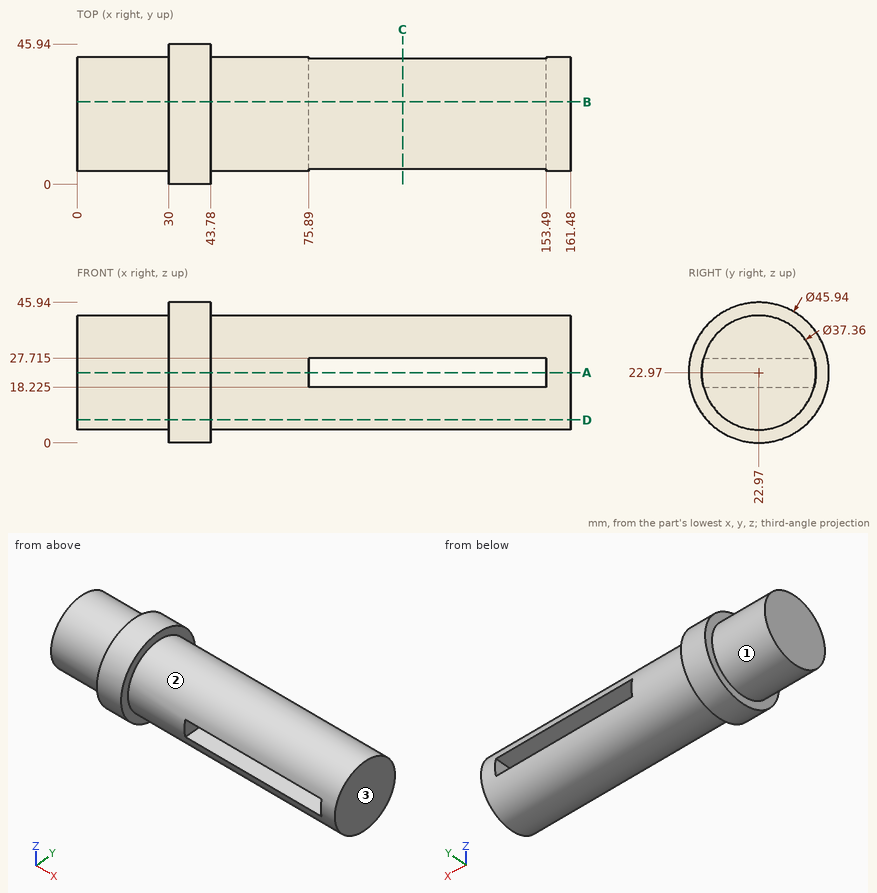
Study the drawing (mm; zero at the part's minimum x, y, z) and answer. A direction names the side the tool comes from. Coordinates: 2 decimals unless noted, no trailing zeros. Write each loop counter-clockwise with the first axis right and the second up, starting at its lowest first coordinate (ties: lowest second). Pieces come first, ordered by that corner, then holes. Notation, with made-up numbers: (38, 24) - (80, 24) arc R14 ccw to (80, 48) - close; hole circle Ø2 at (36, 80.5). An arc over 180 degrees is marked (long way). Answer as a JSON object with one key per item and string values. Group by question number.
1. A cutting plane is placed at C-C (x = 106.5). Determine the outline of the cut face in (y, z) (3 decimals).
2. Consider L1, parallel to X at y = 7.5, z = 19.5; L2, parallel to Z at x = 152, y = 22 (3 decimals); L3, parallel to Z at x = 8, y = 23.5. Determine where each line is inside the solid, lowest interval first. Write a range as [from, to].
3. A cutting plane is placed at B-B (y = 27). Determine the outline of the cut face in (x, z) (3 decimals), plus the area to 3 significant figures.
4. Which of the six approach directions +Z, -Z, +X, -X, +Y, -Y give full straight-line access (tool end or side, diameter ignored) to the marked faces 1, 2 and 3?
5. A cutting plane is placed at A-A (z = 22.97). Determine the outline of the cut face in (x, y), plus the area to 3 significant figures.
6. A cutting plane is placed at D-D (z = 7.5). Determine the outline of the cut face in (x, y), plus the area to 3 significant figures.
7. Each of these flat-tipped pins is pushed along its axis until it touches: P1, Ø3, axis at x = 135.5, z = 11, coming from the +Y side; P2, Ø1, axis at x = 106, y = 24, coming from the -Z side; P3, Ø5, axis at x = 30.5, y = 38, coming from the +Z side. Where does it stop, or does it pass through?
Worked out:
{
 "1": {"outline": "(4.903, 18.225) arc R18.68 ccw to (41.037, 18.225) - close; (4.903, 27.715) - (41.037, 27.715) arc R18.68 ccw to start"},
 "2": {"L1": "x = [0, 75.89], [153.49, 161.48]", "L2": "z = [4.315, 18.225], [27.715, 41.625]", "L3": "z = [4.3, 41.64]"},
 "3": {"outline": "(0, 4.73) - (30, 4.73) - (30, 0.356) - (43.78, 0.356) - (43.78, 4.73) - (161.48, 4.73) - (161.48, 41.21) - (43.78, 41.21) - (43.78, 45.584) - (30, 45.584) - (30, 41.21) - (0, 41.21) - close; hole (75.89, 18.225) - (153.49, 18.225) - (153.49, 27.715) - (75.89, 27.715) - close", "area": "5,270 mm²"},
 "4": {"face 1": "-X", "face 2": "+X", "face 3": "+Z, -Z, +X, +Y, -Y"},
 "5": {"outline": "(0, 4.29) - (30, 4.29) - (30, 0) - (43.78, 0) - (43.78, 4.29) - (75.89, 4.29) - (75.89, 41.65) - (43.78, 41.65) - (43.78, 45.94) - (30, 45.94) - (30, 41.65) - (0, 41.65) - close; (153.49, 4.29) - (161.48, 4.29) - (161.48, 41.65) - (153.49, 41.65) - close", "area": "3,250 mm²"},
 "6": {"outline": "(0, 12.5) - (30, 12.5) - (30, 5.99) - (43.78, 5.99) - (43.78, 12.5) - (161.48, 12.5) - (161.48, 33.44) - (43.78, 33.44) - (43.78, 39.95) - (30, 39.95) - (30, 33.44) - (0, 33.44) - close", "area": "3,560 mm²"},
 "7": {"P1": "stops at y = 38.44", "P2": "stops at z = 4.3", "P3": "stops at z = 42.22"}
}
